Source: CAD feature listing. Evaluate the final solid. Frame: model axes, mm. Face numbers are marked on the shaded views. A direction names the side the tool comes from. Coordinates: 2 decimals unless noted, no trailing zeros. Order: outer loops, then holes, each group sorted by start corner. A loop starts at its lowest first (then second) coordinate and runs counter-clockwise, first axis right, second up.
```python
from build123d import *

# Parameters (mm, degrees)
F1_DEPTH              = 34.2
F2_W                  = 28.2
F2_H                  = 28.2
F3_DEPTH              = 31.2
F4_W                  = 34.2
F4_H                  = 34.2
F5_DEPTH              = 34.2
F6_W                  = 28.2
F6_H                  = 28.2
F7_DEPTH              = 31.2
F10_D                 = 3.3
F10_DEPTH             = 25
F10_CSINK_D           = 6.72
F10_CSINK_ANGLE       = 90
F10_TIP               = 0.9914200214
F10_ON_F9_D           = 3.3
F10_ON_F9_DEPTH       = 25
F10_ON_F9_CSINK_D     = 6.72
F10_ON_F9_CSINK_ANGLE = 90
F10_ON_F9_TIP         = 0.9914200214
F12_D                 = 5.5
F13_R                 = 5
F14_R                 = 1.49999


# Not quite as in the source:
# - a fillet or chamfer is up to 0.001 mm smaller than in the source, because OpenCascade refuses the exact size


with BuildPart() as f1:
    # F0 (on Top) → F1 (new body)
    with BuildSketch(Plane.XY):
        Polygon((-34.2, 0), (-8, 0), (0, 0), (0, 34.2), (-34.2, 34.2), align=None)
        with BuildLine():
            Line((0, 0), (-8, 0))
            Line((-8, 0), (-8, -4))
            ThreePointArc((-8, -4), (-4, -8), (0, -4))
            Line((0, -4), (0, 0))
        make_face()
    extrude(amount=F1_DEPTH)

    # F2 (on face) → F3 (cut)
    with BuildSketch(Plane.XY.offset(34.2)):
        with Locations((-17.1, 17.1)):
            Rectangle(F2_W, F2_H)
    extrude(amount=-F3_DEPTH, mode=Mode.SUBTRACT)

    # F4 (on face) → F5 (join)
    with BuildSketch(Plane(origin=(-34.2, 0, 0), x_dir=(0, -1, 0), z_dir=(-1, 0, 0))):
        with Locations((-17.1, 17.1)):
            Rectangle(F4_W, F4_H)
    extrude(amount=F5_DEPTH)

    # F6 (on face) → F7 (cut)
    with BuildSketch(Plane(origin=(-68.4, 0, 0), x_dir=(0, -1, 0), z_dir=(-1, 0, 0))):
        with Locations((-17.1, 17.1)):
            Rectangle(F6_W, F6_H)
    extrude(amount=-F7_DEPTH, mode=Mode.SUBTRACT)

    # F10
    with Locations(Plane(origin=(0, 34.2, 0), x_dir=(-1, 0, 0), z_dir=(0, 1, 0))):
        with Locations((17.05, 17.1), (51.35, 17.1)):
            CounterSinkHole(F10_D / 2, F10_CSINK_D / 2, depth=F10_DEPTH, counter_sink_angle=F10_CSINK_ANGLE)
            with Locations((0, 0, -(F10_DEPTH + F10_TIP / 2))):  # 118° drill point
                Cone(0, F10_D / 2, F10_TIP, mode=Mode.SUBTRACT)

    # F10 on F9
    with Locations(Plane(origin=(-37.2, 0, 0), x_dir=(0, -1, 0), z_dir=(-1, 0, 0))):
        with Locations((-17.1, 17.1)):
            CounterSinkHole(F10_ON_F9_D / 2, F10_ON_F9_CSINK_D / 2, depth=F10_ON_F9_DEPTH, counter_sink_angle=F10_ON_F9_CSINK_ANGLE)
            with Locations((0, 0, -(F10_ON_F9_DEPTH + F10_ON_F9_TIP / 2))):  # 118° drill point
                Cone(0, F10_ON_F9_D / 2, F10_ON_F9_TIP, mode=Mode.SUBTRACT)

    # F12 (through all)
    with Locations(Plane.XY.offset(34.2)):
        with Locations((-4, -4)):
            Hole(F12_D / 2)

    # F13
    f13_edges = [f1.edges().sort_by_distance(p)[0] for p in [
        (-8, 0, 17.1),
    ]]
    fillet(f13_edges, radius=F13_R)

    # F14 (radius 1.5 in the source; OpenCascade refuses exactly that, so slightly less here)
    f14_edges = [f1.edges().sort_by_distance(p)[0] for p in [
        (-17.1, 3, 34.2),
        (-31.2, 17.1, 34.2),
        (-17.1, 31.2, 34.2),
        (-17.1, 31.2, 3),
        (0, 15.1, 34.2),
        (-40.672136, 0, 34.2),
        (-68.4, 17.1, 34.2),
        (-34.2, 34.2, 34.2),
        (0, 34.2, 17.1),
        (-68.4, 17.1, 31.2),
        (-68.4, 0, 17.1),
        (-68.4, 3, 17.1),
        (-68.4, 31.2, 17.1),
        (-68.4, 34.2, 17.1),
        (-68.4, 17.1, 3),
        (-68.4, 17.1, 0),
        (-40.672136, 0, 0),
        (-34.2, 34.2, 0),
    ]]
    fillet(f14_edges, radius=F14_R)


solid = f1.part
```
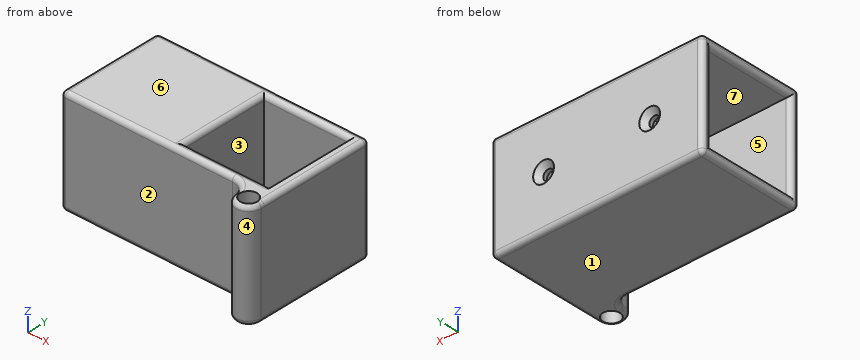
1. Pin query (flat end, axial travel): P1, Ø15.5, axis at y = 18, z = 17.5, coming from the -X side; P2, Ø5.5, axis at x = -17.05, z = 17.1, coming from the +Y side; P3, Ø9.5, axis at x = -52, z = 21, coming from the -Y side; P4, Ø4.5, axis at x = -4, y = -4, coming from the +Z side. Return the tip coordinate at first contact, or that it passes through.
Findings:
P1: stops at x = -37.2
P2: stops at y = 33.59
P3: stops at y = 0
P4: passes through
2. Ray query, line 1 (Y direction, x = -14, z = 5); line 2 (X direction, y = 20, z = 3.5); line 3 (Y direction, x = -4.5, z = 28.5). Return the intervals inside material, ascending.
Findings:
line 1: y = 0 to 3, 31.2 to 34.2
line 2: x = -37.2 to -31.2, -3 to 0
line 3: y = -7.97 to -6.7, -1.3 to 3, 31.2 to 34.2
3. Draft query along Z for the marked faces 4, 5, 6 and 7. Return one class per face: released by +Z, released by -Z, zero draft, split by the parting line, or undercut.
Findings:
face 4: zero draft
face 5: undercut
face 6: released by +Z
face 7: undercut
4. Section query C-C on z = 17.1. Count the separate pieces of the cut face and the enclosed holes in it, plus the area to 3 significant figures.
Findings:
separate pieces: 3
enclosed holes: 1
area: 652 mm2
5. Section query D-D on x = -51.35. Return loops of the section in (y, z), plus the area to 3 significant figures.
Findings:
outline: (0, 1.5) arc R1.5 ccw to (1.5, 0) - (32.7, 0) arc R1.5 ccw to (34.2, 1.5) - (34.2, 13.74) - (32.49, 15.45) - (31.2, 15.45) - (31.2, 3) - (3, 3) - (3, 31.2) - (31.2, 31.2) - (31.2, 18.75) - (32.49, 18.75) - (34.2, 20.46) - (34.2, 32.7) arc R1.5 ccw to (32.7, 34.2) - (1.5, 34.2) arc R1.5 ccw to (0, 32.7) - close
area: 360 mm2
6. Section query B-B on x = -43.5. Return loops of the section in (y, z), plus the area to 3 significant figures.
Findings:
outline: (0, 1.5) arc R1.5 ccw to (1.5, 0) - (32.7, 0) arc R1.5 ccw to (34.2, 1.5) - (34.2, 32.7) arc R1.5 ccw to (32.7, 34.2) - (1.5, 34.2) arc R1.5 ccw to (0, 32.7) - close; hole (3, 3) - (31.2, 3) - (31.2, 31.2) - (3, 31.2) - close
area: 372 mm2
7. Access query for the marked faces 1, 2 and 3. Directions: +Z, -Z, +X, -X, +Y, -Y. A direction counts if a zero-diameter tool reaches every point of the face in a straight line with its end or side. Return the directions, or none.
Findings:
face 1: -Z, +X, -X, +Y, -Y
face 2: +Z, -Z, -X, -Y
face 3: +Z
